CAD build for the part. Positions are in the model's coordinates, mm. Face numbers are marked on the shaded views. A direction names the side the tool comes from. Give positions to 0.01 mm unless a question says otherwise; leave off trailing zeros. Loops run counter-clockwise (first coordinate to the right, second up) from the corner with the lowest first, then second, coordinate; pieces in that order, holes last.
Item 1: Saw through at B-B on y = 4.99. Give the cut face in (x, z).
Item 2: Which spindle directions (+Z, -Z, +X, -X, +Y, -Y) get a long thin tool onto all of the face, cutting with end or side? Do the marked faces 4 and 5. Say none if no direction does.
Item 3: Mould opens along X. For the marked faces 1, 2 and 3 say: released by +X, released by -X, zero draft, split by the parting line, or undercut.
Item 4: Saw through at D-D on z = -30. Give the cut face in (x, y).
Item 5: Saw through at C-C on y = 0. Give the cut face in (x, z), plus the area to 3 significant figures.
Item 6: Saw through at A-A on z = -4. Give the cut face in (x, y), plus the area to 3 significant figures.
Item 7: Drop a flat-ended pin along its axis: P1, Ø10, axis at x = 15, y = -5, coming from the -Z side. Give the stop position or say it passes through.
Item 8: Probe probe 1 along X at (y, z) = (-11, -21); probe 2 along X at (y, z) = (4, 2); probe 3 along Z at (x, y) = (-3, -4.5). List the from-to ranges inside material, lowest first.
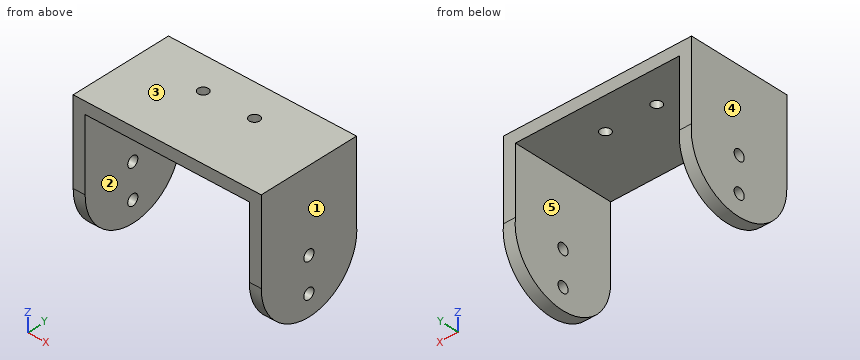
from build123d import *

# Parameters (mm, degrees)
SKETCH_1_W          = 55
SKETCH_1_H          = 30
EXTRUDE_1_DEPTH     = 3.5
SKETCH_2_R          = 1.592723526
EXTRUDE_2_DEPTH     = 3.5
SKETCH_3_R          = 1.5
CUT_EXTRUDE_1_DEPTH = 3.5


with BuildPart() as part:
    # 草图1 → 凸台-拉伸1 (new body)
    with BuildSketch(Plane.XY):
        Rectangle(SKETCH_1_W, SKETCH_1_H)
    extrude(amount=EXTRUDE_1_DEPTH)

    # 草图2 → 凸台-拉伸2 (add)
    with BuildSketch(Plane(origin=(27.5, 0, 0), x_dir=(0, 0, -1), z_dir=(1, 0, 0))):
        with BuildLine():
            Line((0, 15), (0, -15))
            Line((0, -15), (21, -15))
            ThreePointArc((21, -15), (36.119015722, 0.838004237), (19.419767517, 15))
            Line((19.419767517, 15), (0, 15))
        make_face()
        with Locations((20, 0)):
            Circle(SKETCH_2_R, mode=Mode.SUBTRACT)
        with Locations(Location((30, 0, 0), (0, 0, 180))):
            Circle(SKETCH_2_R, mode=Mode.SUBTRACT)
    extrude_2 = extrude(amount=-EXTRUDE_2_DEPTH)

    # 镜向1: 凸台-拉伸2 across plane
    add(extrude_2.mirror(Plane(origin=(0, 0, 0), x_dir=(0, 0, 1), z_dir=(1, 0, 0))))

    # 草图3 → 切除-拉伸1 (cut)
    with BuildSketch(Plane.XY.offset(3.5)):
        with Locations(Location((6.970033691, 4.99, 0), (0, 0, 180))):
            Circle(SKETCH_3_R)
        with Locations(Location((-8.029966309, 4.99, 0), (0, 0, 180))):
            Circle(SKETCH_3_R)
    extrude(amount=-CUT_EXTRUDE_1_DEPTH, mode=Mode.SUBTRACT)


solid = part.part
Results below:
1. outline: (-27.5, -35.3) - (-24, -35.3) - (-24, 0) - (-9.53, 0) - (-9.53, 3.5) - (-27.5, 3.5) - close; (-6.53, 0) - (5.47, 0) - (5.47, 3.5) - (-6.53, 3.5) - close; (8.47, 0) - (24, 0) - (24, -35.3) - (27.5, -35.3) - (27.5, 3.5) - (8.47, 3.5) - close
2. face 4: +Z, -Z, -X, +Y, -Y
2. face 5: -Z, +Y, -Y
3. face 1: released by +X
3. face 2: undercut
3. face 3: zero draft
4. outline: (-27.5, -12.08) - (-24, -12.08) - (-24, -1.59) - (-27.5, -1.59) - close; (-27.5, 1.59) - (-24, 1.59) - (-24, 12.17) - (-27.5, 12.17) - close; (24, -12.08) - (27.5, -12.08) - (27.5, -1.59) - (24, -1.59) - close; (24, 1.59) - (27.5, 1.59) - (27.5, 12.17) - (24, 12.17) - close
5. outline: (-27.5, -36.14) - (-24, -36.14) - (-24, -31.59) - (-27.5, -31.59) - close; (-27.5, -28.41) - (-24, -28.41) - (-24, -21.59) - (-27.5, -21.59) - close; (-27.5, -18.41) - (-24, -18.41) - (-24, 0) - (24, 0) - (24, -18.41) - (27.5, -18.41) - (27.5, 3.5) - (-27.5, 3.5) - close; (24, -36.14) - (27.5, -36.14) - (27.5, -31.59) - (24, -31.59) - close; (24, -28.41) - (27.5, -28.41) - (27.5, -21.59) - (24, -21.59) - close
5. area: 401 mm2
6. outline: (-27.5, -15) - (-24, -15) - (-24, 15) - (-27.5, 15) - close; (24, -15) - (27.5, -15) - (27.5, 15) - (24, 15) - close
6. area: 210 mm2
7. P1: stops at z = 0
8. probe 1: x = -27.5 to -24, 24 to 27.5
8. probe 2: x = -27.5 to -9.16, -6.9 to 5.84, 8.1 to 27.5
8. probe 3: z = 0 to 3.5
